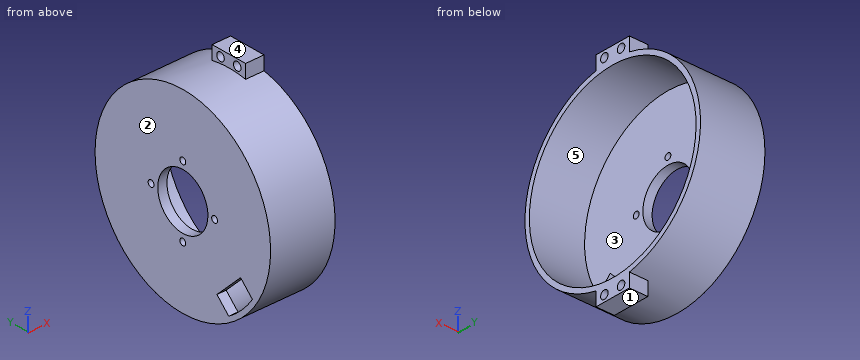
Autodesk Inventor part; units mm, degrees
ref_plane "YZ Plane" through (0, 0, 0) normal (1, 0, 0) x (0, 1, 0)
ref_plane "XZ Plane" through (0, 0, 0) normal (0, 1, 0) x (-1, 0, 0)
ref_plane "XY Plane" through (0, 0, 0) normal (0, 0, 1) x (1, 0, 0)
sketch "Sketch1" plane through (0, 0, 0) normal (1, 0, 0) x (0, 1, 0)
  circle A0 centre (0, 0) radius 19
  circle A1 centre (0, -19) radius 1.75
  circle A2 centre (19, 0) radius 1.75
  circle A3 centre (0, 19) radius 1.75
  circle A4 centre (-19, 0) radius 1.75
  circle A5 centre (0, 0) radius 52.5
  circle A6 centre (0, 0) radius 40
  dimension "d0" = 38
  dimension "d1" = 3.5
  dimension "d4" = 360
  dimension "d6" = 105
  dimension "d7" = 80
extrude "Extrusion1" add sketch "Sketch1" along normal blind 5 contours A2 A0 A1 A4 A3 | A5 | A6
sketch "Sketch2" plane through (0, 0, 0) normal (-1, 0, 0) x (0, 0, 1)
  circle A0 centre (0, 0) radius 52.5
  circle A1 centre (0, 0) radius 49.875
  dimension "d10" = 105
extrude "Extrusion2" add sketch "Sketch2" against normal blind 35
sketch "Sketch3" plane through (35, 0, 0) normal (1, 0, 0) x (0, 0, -1)
  circle A0 centre (0, 0) radius 52.5
  circle A1 centre (0, 0) radius 47.5
  line L0 (-48.9952, 10) -> (-58.9952, 10)
  line L1 (-58.9952, 10) -> (-58.9952, -10)
  line L2 (-58.9952, -10) -> (-51.5388, -10)
  line L3 (-48.9952, 10) -> (-51.5388, 10)
  line L4 (-47.5, 0) -> (-55.5093, 0)
  line L5 (-55.5093, 0) -> (-55.5093, 5)
  circle A2 centre (-55.5093, 5) radius 2.25
  line L6 (-55.5093, 0) -> (-55.5093, -5)
  circle A3 centre (-55.5093, -5) radius 2.25
  line L7 (48.9952, -10) -> (58.9952, -10)
  line L8 (58.9952, -10) -> (58.9952, 10)
  line L9 (58.9952, 10) -> (51.5388, 10)
  line L10 (48.9952, -10) -> (51.5388, -10)
  line L11 (47.5, 0) -> (55.5093, 0)
  line L12 (55.5093, 0) -> (55.5093, -5)
  circle A4 centre (55.5093, -5) radius 2.25
  line L13 (55.5093, 0) -> (55.5093, 5)
  circle A5 centre (55.5093, 5) radius 2.25
  point P0 (51.5388, -10)
  point P1 (47.2562, -4.8066)
  point P2 (47.2562, 4.8066)
  point P3 (51.5388, -10)
  point P4 (-47.2562, 4.8066)
  point P5 (-47.2562, -4.8066)
  dimension "d14" = 10
  dimension "d15" = 20
  dimension "d17" = 5
  dimension "d18" = 4.5
  dimension "d19" = 5
  dimension "d20" = 4.5
  dimension "d23" = 360
  dimension "d33" = 105
extrude "Extrusion3" add sketch "Sketch3" against normal blind 10 contours A0 L9 L8 L7 | A0 L2 L1 L0
sketch "Sketch4" plane through (5, 0, 0) normal (1, 0, 0) x (0, 0, -1)
  circle A0 centre (0, 0) radius 15
  line L0 (0, 0) -> (7.0711, 7.0711)
  line L1 (0, 0) -> (10, 0) construction
  line L2 (7.0711, 7.0711) -> (41.6219, -27.4797)
  circle A1 centre (0, 0) radius 49.875
  line L3 (0, 0) -> (-7.0711, -7.0711)
  line L4 (-7.0711, -7.0711) -> (27.4797, -41.6219)
  line L5 (41.6219, -27.4797) -> (34.5508, -20.4087)
  line L6 (34.5508, -20.4087) -> (20.4087, -34.5508)
  point P0 (0.8346, -14.9768)
  point P1 (14.9768, -0.8346)
  point P2 (48.8622, 10)
  point P3 (-48.8622, 10)
  dimension "d27" = 30
  dimension "d28" = 10
  dimension "d29" = 45
  dimension "d30" = 10
  dimension "d34" = 10
extrude "Extrusion4" cut sketch "Sketch4" against normal blind 10 contours A0 L2 L0 L3 L4 | L4 L3 L0 L2 A0 | L6 L2 A1 L4
equation "\"BendRadius\" = Thickness"
equation "\"BendReliefWidth\" = Thickness"
equation "\"BendReliefDepth\" = 0.5 * Thickness"
equation "\"CornerReliefSize\" = 4 * Thickness"
equation "\"MinimumRemnant\" = 2 * Thickness"
equation "\"TransitionRadius\" = BendRadius"
equation "\"JacobiRadiusSize\" = BendRadius"
equation "\"GapSize\" = Thickness"
properties part number "MotorHouse"
Part model, mm, in its own coordinate system. Face numbers are marked on the shaded views. A direction names the side the tool comes from. Give positions to 0.01 mm unless a question says otherwise; leave off trailing zeros. Order: outer loops, then holes, each group sorted by start corner. A loop starts at its lowest first (then second) coordinate and runs counter-clockwise, first axis right, second up. Notation, with made-up numbers: (89.25, 33.25) - (101.25, 33.25) arc R20 ccw to (101.25, 37.25) - close; hole circle Ø5 at (24.25, -9). An arc over 180 degrees is marked (long way). One line per question, with ' | ' between items.
1. Drill centre lines: probe 1 along Z at (x, y) = (3.75, 0); probe 2 along Z at (x, y) = (31, -5); probe 3 along Y at (x, z) = (1, -19). Where is each one in solid material? Low to high.
Filled in:
probe 1: -52.5 to -20.75, -17.25 to -15, 15 to 17.25, 20.75 to 52.5 | probe 2: -59 to -57.76, -53.26 to -49.62, 49.62 to 53.26, 57.76 to 59 | probe 3: -48.94 to -1.75, 1.75 to 48.94
2. Band-saw the part on B-B on x = 20.5. List the corners of the cut face in (y, z) (3 decimals).
Filled in:
outline: circle Ø105 at (0, 0); hole circle Ø99.75 at (0, 0)
3. Drop flat-ended pins along their axis: P1, Ø3, axis at y = 0, z = 19, coming from the -X side; P2, Ø6, axis at y = 5, z = -55.51, coming from the -X side; P3, Ø1, axis at y = 19, z = -45, coming from the +X side; P4, Ø2, axis at y = -25, z = 9, coming from the -X side. Give the stop position or say it passes through.
Filled in:
P1: through | P2: x = 25 | P3: x = 5 | P4: x = 0
4. Which spindle directions (+Z, -Z, +X, -X, +Y, -Y) get a long thin tool onto all of the face, cutting with end or side? Do the marked faces 4 and 5. Say none if no direction does.
Filled in:
face 4: +Z, +X, -X, +Y, -Y | face 5: +X
5. Pull direction X, two halves, no side cores. Call the marked faces 1, 2 and 3: +X half, -X half, draft (parallel to the pull), parting line (faces both ways), or undercut.
Filled in:
face 1: draft | face 2: -X half | face 3: +X half
6. Band-saw the part on A-A on z = -9. List the corners of the cut face in (x, y).
Filled in:
outline: (0, -51.72) - (35, -51.72) - (35, -49.06) - (5, -49.06) - (5, -12) - (0, -12) - close; (0, 12) - (5, 12) - (5, 49.06) - (35, 49.06) - (35, 51.72) - (0, 51.72) - close
